Geometry check sheet. Reference: the model listing, model coordinates, mm. Coordinates: 2 decimals unless noted, no trailing zeros. Write each question's results on one line, items separated by ' | '. Start each with the question number.
(1) Sectioned sample at A-A (z = 558). State how many separate pieces and enclosed holes the cut face has, plus the area to 3 significant figures.
(2) Go/stop test with flat-tipped pins: pin 1 Ø0.6 at (x, z) = (-9.5, 398) entering from +Y; pin 2 Ø0.7 at (y, z) = (22, 246.5) entering from +X; pin 3 Ø2.5 at (y, z) = (-2, 388) entering from +X. Record where each tip stops, or that it passes through.
(3) Material ranges on probe 1 along X at (y, z) = (5, 503); probe 2 along Y at (x, z) = (6.5, 50); probe 3 along Y at (x, z) = (0, 233.5), recorded low to high.
from build123d import *

# Parameters (mm, degrees)
SKETCH_30_R     = 2.5
EXTRUDE_3_DEPTH = 600


with BuildPart() as part:
    # 草图30 → 凸台-拉伸3 (new body)
    with BuildSketch(Plane.XY):
        with BuildLine():
            Line((-8.1, 14.5), (-8.1, 16.9))
            Line((-8.1, 16.9), (-9.5, 16.9))
            Line((-9.5, 16.9), (-9.5, 16.4))
            Line((-9.5, 16.4), (-10, 16.4))
            Line((-10, 16.4), (-10, 3.6))
            Line((-10, 3.6), (-9.5, 3.6))
            Line((-9.5, 3.6), (-9.5, 3.1))
            Line((-9.5, 3.1), (-8.1, 3.1))
            Line((-8.1, 3.1), (-8.1, 5.5))
            Line((-8.1, 5.5), (-6.489949494, 5.5))
            Line((-6.489949494, 5.5), (-3.9, 2.910050506))
            Line((-3.9, 2.910050506), (-3.9, 0.519615242))
            Line((-3.9, 0.519615242), (-3.6, 0))
            Line((-3.6, 0), (-3.9, -0.519615242))
            Line((-3.9, -0.519615242), (-3.9, -2.910050506))
            Line((-3.9, -2.910050506), (-6.489949494, -5.5))
            Line((-6.489949494, -5.5), (-8.1, -5.5))
            Line((-8.1, -5.5), (-8.1, -3.1))
            Line((-8.1, -3.1), (-9.5, -3.1))
            Line((-9.5, -3.1), (-9.5, -3.6))
            Line((-9.5, -3.6), (-10, -3.6))
            Line((-10, -3.6), (-10, -8.5))
            ThreePointArc((-10, -8.5), (-9.560660172, -9.560660172), (-8.5, -10))
            Line((-8.5, -10), (-3.6, -10))
            Line((-3.6, -10), (-3.6, -9.5))
            Line((-3.6, -9.5), (-3.1, -9.5))
            Line((-3.1, -9.5), (-3.1, -8.1))
            Line((-3.1, -8.1), (-5.5, -8.1))
            Line((-5.5, -8.1), (-5.5, -6.489949494))
            Line((-5.5, -6.489949494), (-2.910050506, -3.9))
            Line((-2.910050506, -3.9), (-0.519615242, -3.9))
            Line((-0.519615242, -3.9), (0, -3.6))
            Line((0, -3.6), (0.519615242, -3.9))
            Line((0.519615242, -3.9), (2.910050506, -3.9))
            Line((2.910050506, -3.9), (5.5, -6.489949494))
            Line((5.5, -6.489949494), (5.5, -8.1))
            Line((5.5, -8.1), (3.1, -8.1))
            Line((3.1, -8.1), (3.1, -9.5))
            Line((3.1, -9.5), (3.6, -9.5))
            Line((3.6, -9.5), (3.6, -10))
            Line((3.6, -10), (8.5, -10))
            ThreePointArc((8.5, -10), (9.560660172, -9.560660172), (10, -8.5))
            Line((10, -8.5), (10, -3.6))
            Line((10, -3.6), (9.5, -3.6))
            Line((9.5, -3.6), (9.5, -3.1))
            Line((9.5, -3.1), (8.1, -3.1))
            Line((8.1, -3.1), (8.1, -5.5))
            Line((8.1, -5.5), (6.489949494, -5.5))
            Line((6.489949494, -5.5), (3.9, -2.910050506))
            Line((3.9, -2.910050506), (3.9, -0.519615242))
            Line((3.9, -0.519615242), (3.6, 0))
            Line((3.6, 0), (3.9, 0.519615242))
            Line((3.9, 0.519615242), (3.9, 2.910050506))
            Line((3.9, 2.910050506), (6.489949494, 5.5))
            Line((6.489949494, 5.5), (8.1, 5.5))
            Line((8.1, 5.5), (8.1, 3.1))
            Line((8.1, 3.1), (9.5, 3.1))
            Line((9.5, 3.1), (9.5, 3.6))
            Line((9.5, 3.6), (10, 3.6))
            Line((10, 3.6), (10, 16.4))
            Line((10, 16.4), (9.5, 16.4))
            Line((9.5, 16.4), (9.5, 16.9))
            Line((9.5, 16.9), (8.1, 16.9))
            Line((8.1, 16.9), (8.1, 14.5))
            Line((8.1, 14.5), (6.489949494, 14.5))
            Line((6.489949494, 14.5), (3.9, 17.089949494))
            Line((3.9, 17.089949494), (3.9, 19.480384758))
            Line((3.9, 19.480384758), (3.6, 20))
            Line((3.6, 20), (3.9, 20.519615242))
            Line((3.9, 20.519615242), (3.9, 22.910050506))
            Line((3.9, 22.910050506), (6.489949494, 25.5))
            Line((6.489949494, 25.5), (8.1, 25.5))
            Line((8.1, 25.5), (8.1, 23.1))
            Line((8.1, 23.1), (9.5, 23.1))
            Line((9.5, 23.1), (9.5, 23.6))
            Line((9.5, 23.6), (10, 23.6))
            Line((10, 23.6), (10, 28.5))
            ThreePointArc((10, 28.5), (9.560660172, 29.560660172), (8.5, 30))
            Line((8.5, 30), (3.6, 30))
            Line((3.6, 30), (3.6, 29.5))
            Line((3.6, 29.5), (3.1, 29.5))
            Line((3.1, 29.5), (3.1, 28.1))
            Line((3.1, 28.1), (5.5, 28.1))
            Line((5.5, 28.1), (5.5, 26.489949494))
            Line((5.5, 26.489949494), (2.910050506, 23.9))
            Line((2.910050506, 23.9), (0.519615242, 23.9))
            Line((0.519615242, 23.9), (0, 23.6))
            Line((0, 23.6), (-0.519615242, 23.9))
            Line((-0.519615242, 23.9), (-2.910050506, 23.9))
            Line((-2.910050506, 23.9), (-5.5, 26.489949494))
            Line((-5.5, 26.489949494), (-5.5, 28.1))
            Line((-5.5, 28.1), (-3.1, 28.1))
            Line((-3.1, 28.1), (-3.1, 29.5))
            Line((-3.1, 29.5), (-3.6, 29.5))
            Line((-3.6, 29.5), (-3.6, 30))
            Line((-3.6, 30), (-8.5, 30))
            ThreePointArc((-8.5, 30), (-9.560660172, 29.560660172), (-10, 28.5))
            Line((-10, 28.5), (-10, 23.6))
            Line((-10, 23.6), (-9.5, 23.6))
            Line((-9.5, 23.6), (-9.5, 23.1))
            Line((-9.5, 23.1), (-8.1, 23.1))
            Line((-8.1, 23.1), (-8.1, 25.5))
            Line((-8.1, 25.5), (-6.489949494, 25.5))
            Line((-6.489949494, 25.5), (-3.9, 22.910050506))
            Line((-3.9, 22.910050506), (-3.9, 20.519615242))
            Line((-3.9, 20.519615242), (-3.6, 20))
            Line((-3.6, 20), (-3.9, 19.480384758))
            Line((-3.9, 19.480384758), (-3.9, 17.089949494))
            Line((-3.9, 17.089949494), (-6.489949494, 14.5))
            Line((-6.489949494, 14.5), (-8.1, 14.5))
        make_face()
        with Locations((0, 20)):
            Circle(SKETCH_30_R, mode=Mode.SUBTRACT)
        Circle(SKETCH_30_R, mode=Mode.SUBTRACT)
        Polygon((5.910050506, 6.9), (2.910050506, 3.9), (-2.910050506, 3.9), (-5.910050506, 6.9), (-8, 6.9), (-8, 13.1), (-5.910050506, 13.1), (-2.910050506, 16.1), (2.910050506, 16.1), (5.910050506, 13.1), (8, 13.1), (8, 6.9), align=None, mode=Mode.SUBTRACT)
    extrude(amount=EXTRUDE_3_DEPTH)


solid = part.part
Outcome:
1) separate pieces: 1 | enclosed holes: 3 | area: 295 mm2
2) pin 1: stops at y = 29.83 | pin 2: stops at x = 3.9 | pin 3: stops at x = 9.5
3) probe 1: x = -10 to -8.1, -5.99 to -4.01, 4.01 to 5.99, 8.1 to 10 | probe 2: y = -10 to -5.5, 5.5 to 6.9, 13.1 to 14.5, 25.5 to 30 | probe 3: y = -3.6 to -2.5, 2.5 to 3.9, 16.1 to 17.5, 22.5 to 23.6
